Read the model definition and answer for the solid it produces. Units are mm, in the model's axes. A direction names the side the tool comes from. Coordinates: 2 decimals unless noted, no trailing zeros. Loops run counter-clockwise (first coordinate to the right, second up) from the corner with the lowest first, then second, coordinate; pieces in that order, holes last. Notation, with made-up numbers: M 79.5,18.25 L 121.5,18.25 A7 ccw 121.5,22.25 Z; hole C 34,-25.5 d5. An arc over 180 degrees is marked long. Use one line per item in the form item = value. Start each with the question number.
1. The part is cut by section C-C (z = -6.5). Give the vertices of the cut face in (x, y).
2. Find the intervals of material crossed by probe 1 along Y at (x, z) = (0, -7.95); probe 2 along X at (y, z) = (-12, -3.5); probe 3 along Y at (x, z) = (1, -2), in increasing order. Write a range as [from, to].
3. For a pull along Y with two mould halves and no side action, classify faces 1 (the cylindrical face through (-8.67, -39.05, -4.93)), 2 (the cylindrical face through (-5.689, 34.585, -5.07)), 3 (the flat face through (17.2, -17.2, 0)) as released by +Y, released by -Y, zero draft, split by the parting line, or undercut.
4. A tool of negligible diameter and unlimited length cuts with its end or side. For faces 4 (the flat face through (10, -5, -4)), 5 (the cylindrical face through (27.3, -11.64, -5.07)), from which of +Z, -Z, +X, -X, +Y, -Y can it reach the whole face along a straight path? Write none if from no direction.
5. Flat-ended cylindrical pins translate along their axes: pin 1 (1 mm diameter, centred on y = -22, z = -6, fed in from -X); pin 2 (1 mm diameter, centred on y = 26.5, z = -2.5, fed in from -X); pin 3 (8 mm diameter, centred on x = 0.5, y = -12.5, fed in from +Z). Find the tip coordinate at first contact, or state that the pin passes through.
6. The part is cut by section D-D (x = 13). Give the vertices of the cut face in (y, z), plus the area to 3 significant figures.
7. The part is cut by section A-A (y = 0). Give the vertices of the cut face in (x, z), plus the area to 3 significant figures.
from build123d import *

# Parameters (mm, degrees)
F0_R          = 40
F1_DEPTH      = 10
F2_R          = 24
F3_DEPTH      = 4
F3_DEPTH_BACK = 10
F6_D          = 21
F7_D          = 6.4


with BuildPart() as f1:
    # F0 (on Top) → F1 (new body)
    with BuildSketch(Plane.XY):
        Circle(F0_R)
    extrude(amount=-F1_DEPTH)

    # F2 (on Top) → F3 (cut, two sides)
    with BuildSketch(Plane.XY) as f3_sk:
        Circle(F2_R)
    extrude(amount=-F3_DEPTH, mode=Mode.SUBTRACT)
    extrude(f3_sk.sketch, amount=F3_DEPTH_BACK, mode=Mode.SUBTRACT)

    # F6 (through all)
    with Locations(Plane.XY.offset(-4)):
        with Locations((0, 0)):
            Hole(F6_D / 2)

    # F7 (through all)
    with Locations(Plane.XY):
        with Locations((-6.105887852, 31.4120698703), (24.1507065671, 20.9938889277), (30.2565944192, -10.4181809426), (6.105887852, -31.4120698703), (-24.1507065671, -20.9938889277), (-30.2565944192, 10.4181809426)):
            Hole(F7_D / 2)


solid = f1.part
Computed values:
q1.outline = C 0,0 d80; hole C -30.26,10.42 d6.4; hole C -24.15,-20.99 d6.4; hole C 0,0 d21; hole C -6.11,31.41 d6.4; hole C 6.11,-31.41 d6.4; hole C 24.15,20.99 d6.4; hole C 30.26,-10.42 d6.4
q2.probe_1 = [-40, -10.5], [10.5, 40]
q2.probe_2 = [-38.16, -20.78], [20.78, 27.47], [33.04, 38.16]
q2.probe_3 = [-39.99, -23.98], [23.98, 39.99]
q3.face_1 = split by the parting line
q3.face_2 = undercut
q3.face_3 = zero draft
q4.face_4 = +Z
q4.face_5 = +Z, -Z
q5.pin_1 = -33.73
q5.pin_2 = -30.4
q5.pin_3 = -4
q6.outline = M -37.83,-10 L 37.83,-10 L 37.83,0 L 20.17,0 L 20.17,-4 L -20.17,-4 L -20.17,0 L -37.83,0 Z
q6.area = 595 mm²
q7.outline = M -40,-10 L -10.5,-10 L -10.5,-4 L -24,-4 L -24,0 L -40,0 Z; M 10.5,-10 L 40,-10 L 40,0 L 24,0 L 24,-4 L 10.5,-4 Z
q7.area = 482 mm²
